from build123d import *

# Parameters (mm, degrees)
BOSS_EXTRU_1_DEPTH      = 250
ENL_V_MAT_EXTRU_1_DEPTH = 16
D_GAGEMENT_M31_D        = 3.2
ESQUISSE6_R             = 5
BOSS_EXTRU_2_DEPTH      = 41.23


with BuildPart() as part:
    # Esquisse1 → Boss.-Extru.1 (new body)
    with BuildSketch(Plane.XY):
        with BuildLine():
            Line((0, 5), (0, 48))
            ThreePointArc((0, 48), (1.464466094, 51.535533906), (5, 53))
            Line((5, 53), (15, 53))
            Line((15, 53), (15, 52))
            Line((15, 52), (5, 52))
            ThreePointArc((5, 52), (2.171572875, 50.828427125), (1, 48))
            Line((1, 48), (1, 5))
            ThreePointArc((1, 5), (2.171572875, 2.171572875), (5, 1))
            Line((5, 1), (15, 1))
            Line((15, 1), (15, 0))
            Line((15, 0), (5, 0))
            ThreePointArc((5, 0), (1.464466094, 1.464466094), (0, 5))
        make_face()
    extrude(amount=BOSS_EXTRU_1_DEPTH)

    # Esquisse5 → Enlèv. mat.-Extru.1 (cut, through all)
    with BuildSketch(Plane.ZY):
        with BuildLine():
            Line((0, 8.142135624), (0, -1))
            Line((0, -1), (21.071067812, -1))
            Line((21.071067812, -1), (21.071067812, 0))
            Line((21.071067812, 0), (8.142135624, 0))
            ThreePointArc((8.142135624, 0), (6.611401894, 0.30448187), (5.313708499, 1.171572875))
            Line((5.313708499, 1.171572875), (1.171572875, 5.313708499))
            ThreePointArc((1.171572875, 5.313708499), (0.30448187, 6.611401894), (0, 8.142135624))
        make_face()
        with BuildLine():
            Line((8.142135624, 53), (21.071067812, 53))
            Line((21.071067812, 53), (21.071067812, 54))
            Line((21.071067812, 54), (0, 54))
            Line((0, 54), (0, 44.857864376))
            ThreePointArc((0, 44.857864376), (0.30448187, 46.388598106), (1.171572875, 47.686291501))
            Line((1.171572875, 47.686291501), (5.313708499, 51.828427125))
            ThreePointArc((5.313708499, 51.828427125), (6.611401894, 52.69551813), (8.142135624, 53))
        make_face()
    enl_v_mat_extru_1 = extrude(amount=-ENL_V_MAT_EXTRU_1_DEPTH, mode=Mode.SUBTRACT)

    # Symétrie1: Enlèv. mat.-Extru.1 across plane
    add(enl_v_mat_extru_1.mirror(Plane(origin=(0, 0, 125), x_dir=(1, 0, 0), z_dir=(0, 0, -1))), mode=Mode.SUBTRACT)

    # Dégagement M31 (through all)
    with Locations(Plane(origin=(0, 53, 0), x_dir=(1, 0, 0), z_dir=(0, 1, 0))):
        with Locations((10, -43.5), (10, -206.5)):
            Hole(D_GAGEMENT_M31_D / 2)

    # Esquisse6 → Boss.-Extru.2 (add)
    with BuildSketch(Plane.ZY):
        with Locations((27.5, 26.5)):
            Circle(ESQUISSE6_R)
        with Locations((222.5, 26.5)):
            Circle(ESQUISSE6_R)
    extrude(amount=BOSS_EXTRU_2_DEPTH)


solid = part.part
Build history of the part. All positions in model axes, mm. A direction names the side the tool comes from. Round coordinates to 2 decimals unless told otherwise and drop trailing zeros. Write each loop counter-clockwise with the first axis right and the second up, starting at its lowest first coordinate (ties: lowest second). Pieces come first, ordered by that corner, then holes. Notation, with made-up numbers: M -34.75,-38.75 L 2.25,-38.75 A8 ccw 2.25,-29.75 Z; hole C 46.25,84 d9. An arc over 180 degrees is marked long. Answer as a JSON object with one key per item and string values. Group by question number.
(1) Cut at B-B (y = 26.5). Give the cut face in (x, z), and give its area (3 significant figures).
(2) Cut at D-D (z = 83). Give the cut face in (x, y).
(3) Drill centre lines: L1, parallel to Z at x = 10, y = 0.5; L2, parallel to Z at x = 10, y = 52.25; L3, parallel to Y at x = 8.5, z = 204. Where is each one in solid material? Low to high.
(4) Cut at C-C (x = -30.5). Give the cut face in (y, z).
(5) Which spindle directions (+Z, -Z, +X, -X, +Y, -Y) get a long thin tool onto all of the face, cutting with end or side? Do faces 1 (the cylindrical face through (-20.33, 28, 227.27)), 2 (the flat face through (1, 27, 123)), 3 (the cylindrical face through (2, 1, 123)). Say none if no direction does.
(6) Flat gauge pins, fed straight in: pin 1 (2.5 mm diameter, centred on x = 10, z = 206.5, fed in from +Y); pin 2 (3.5 mm diameter, centred on x = 10, z = 206.5, fed in from -Y); pin 3 (8 mm diameter, centred on y = 17, z = 170.5, fed in from -X); pin 4 (13 mm diameter, centred on y = 35.5, z = 111.5, fed in from +X). Where does each tip first touch, or does it go through?
(7) Cut at A-A (z = 222.5). Give the cut face in (x, y), and give its area (3 significant figures).
(8) Mould opens along Z. For faces 4 (the cylindrical face through (2.141, 2.203, 123.271)), 5 (the flat face through (0, 26, 123)), 6 (the flat face through (1.058, 49.901, 3.386)) say: pulls with the +Z half, pulls with the -Z half, needs draft (parallel to the pull), parting line crosses it, or undercut.
Responses:
{
 "1": {"outline": "M -41.23,22.5 L 0,22.5 L 0,0 L 1,0 L 1,250 L 0,250 L 0,227.5 L -41.23,227.5 L -41.23,217.5 L 0,217.5 L 0,32.5 L -41.23,32.5 Z", "area": "1,070 mm2"},
 "2": {"outline": "M 0,5 A5 ccw 5,0 L 15,0 L 15,1 L 5,1 A4 cw 1,5 L 1,48 A4 cw 5,52 L 15,52 L 15,53 L 5,53 A5 ccw 0,48 Z"},
 "3": {"L1": "z = 6.21 to 41.9, 45.1 to 204.9, 208.1 to 243.79", "L2": "z = 5.81 to 41.9, 45.1 to 204.9, 208.1 to 244.19", "L3": "y = 0 to 1, 52 to 53"},
 "4": {"outline": "C 26.5,27.5 d10; C 26.5,222.5 d10"},
 "5": {"face 1": "-X", "face 2": "+Z, -Z, +X", "face 3": "+Z, -Z, -X, -Y"},
 "6": {"pin 1": "passes through", "pin 2": "stops at y = 0", "pin 3": "stops at x = 0", "pin 4": "stops at x = 1"},
 "7": {"outline": "M -41.23,21.5 L 0,21.5 L 0,5 A5 ccw 5,0 L 15,0 L 15,1 L 5,1 A4 cw 1,5 L 1,48 A4 cw 5,52 L 15,52 L 15,53 L 5,53 A5 ccw 0,48 L 0,31.5 L -41.23,31.5 Z", "area": "489 mm2"},
 "8": {"face 4": "needs draft", "face 5": "undercut", "face 6": "pulls with the -Z half"}
}
